Build history of the part. All positions in model axes, mm. Face numbers are marked on the shaded views. A direction names the side the tool comes from. Coordinates: 2 decimals unless noted, no trailing zeros. Write each loop counter-clockwise with the first axis right and the second up, starting at its lowest first coordinate (ties: lowest second). Pieces come first, ordered by that corner, then holes.
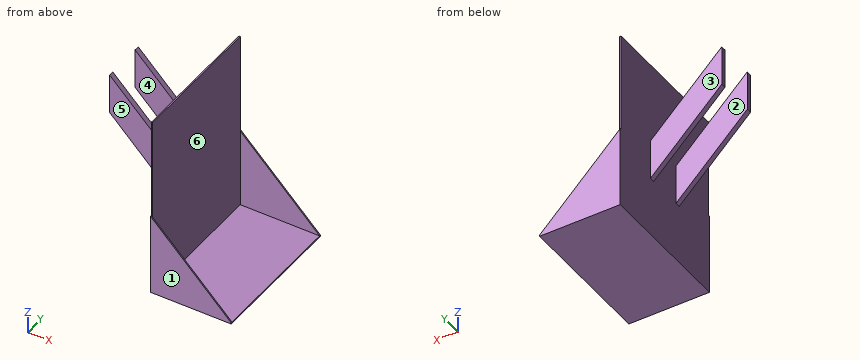
```python
from build123d import *

# Parameters (mm, degrees)
F0_W     = 101.6
F0_H     = 177.8
F1_DEPTH = 1.5875
F3_DEPTH = 1.5875
F5_DEPTH = 1.5875
F7_DEPTH = 1.5875
F8_W     = 6.35
F8_H     = 50.8


with BuildPart() as f1:
    # F0 (on Top) → F1 (new body)
    with BuildSketch(Plane.XY):
        with Locations((50.8, 88.9)):
            Rectangle(F0_W, F0_H)
    extrude(amount=F1_DEPTH)

    # F2 (on Front) → F3 (join)
    with BuildSketch(Plane.XZ):
        Polygon((0, 103.1875), (0, 1.5875), (101.6, 1.5875), align=None)
    extrude(amount=-F3_DEPTH)

    # F4 (on face) → F5 (join)
    with BuildSketch(Plane(origin=(0, 177.8, 0), x_dir=(-1, 0, 0), z_dir=(0, 1, 0))):
        Polygon((-101.6, 1.5875), (0, 1.5875), (0, 103.1875), align=None)
    extrude(amount=-F5_DEPTH)

    # F6 (on face) → F7 (join)
    with BuildSketch(Plane(origin=(0, 0, 0), x_dir=(0, -1, 0), z_dir=(-1, 0, 0))):
        Polygon((-176.2125, 1.5875), (-1.5875, 1.5875), (-1.5875, 103.1875), (-1.5875, 230.1875), (-176.2125, 230.1875), (-176.2125, 103.1875), align=None)
    extrude(amount=-F7_DEPTH)

    # F11: sweep along a path in F10
    with BuildLine(Plane(origin=(0, 66.675, 0), x_dir=(-1, 0, 0), z_dir=(0, 1, 0))) as f11_path:
        Line((0, 76.2), (89.8025612107, 166.0025612107))
    # F8 (on face) → F11 (sweep)
    with BuildSketch(Plane(origin=(0, 0, 0), x_dir=(0, -1, 0), z_dir=(-1, 0, 0))):
        with Locations((-63.5, 101.6)):
            Rectangle(F8_W, F8_H)
        with Locations((-114.3, 101.6)):
            Rectangle(F8_W, F8_H)
    sweep(path=f11_path.line)


solid = f1.part
```
1. Saw through at C-C on y = 16. List the corners of the cut face in (x, z).
Computed values:
outline: (0, 0) - (101.6, 0) - (101.6, 1.59) - (1.59, 1.59) - (1.59, 230.19) - (0, 230.19) - close
2. 3-axis set-ups, long thin cutter, end or side, ignore diameter. For the marked faces 4, 5 and 6: which of +Z, -Z, +X, -X, +Y, -Y reach the whole face in a straight line?
Computed values:
face 4: +Z, -Z, -X
face 5: +Z, -Z, -X, -Y
face 6: +Z, +X
3. Saw through at A-A on z = 133. List the corners of the cut face in (x, y) (1 decimal), plus the area to 3 significant figures.
Computed values:
outline: (-56.8, 60.3) - (-6, 60.3) - (-6, 66.7) - (-56.8, 66.7) - close; (-56.8, 111.1) - (-6, 111.1) - (-6, 117.5) - (-56.8, 117.5) - close; (0, 1.6) - (1.6, 1.6) - (1.6, 176.2) - (0, 176.2) - close
area: 922 mm2
4. Flat gauge pins, fed straight in: pin 1 (1 mm diameter, centred on y = 137.5, z = 80, fed in from -X); pin 2 (5 mm diameter, centred on x = -50.5, z = 164.5, fed in from -Y) (3 decimals); pin 3 (0.5 mm diameter, centred on x = 0.5, z = 143.5, fed in from -Y). Where does each tip first touch, or does it go through?
Computed values:
pin 1: stops at x = 0
pin 2: stops at y = 60.325
pin 3: stops at y = 1.59
5. Saw through at D-D on z = 209.5. List the corners of the cut face in (x, y) (1 decimal).
Computed values:
outline: (-89.8, 60.3) - (-82.5, 60.3) - (-82.5, 66.7) - (-89.8, 66.7) - close; (-89.8, 111.1) - (-82.5, 111.1) - (-82.5, 117.5) - (-89.8, 117.5) - close; (0, 1.6) - (1.6, 1.6) - (1.6, 176.2) - (0, 176.2) - close
6. Mould opens along Y. For the marked faces 1, 2 and 3 say: +Y half, -Y half, draft (parallel to the pull), parting line (faces both ways), or undercut.
Computed values:
face 1: -Y half
face 2: undercut
face 3: +Y half
7. Probe line 1 along Y through (x, z) = (24, 75); line 2 along Y through (x, z) = (-31, 117.5) (3 decimals); line 3 along X through (y, z) = (14, 100). List the from-to ranges inside material, lowest first.
Computed values:
line 1: y = 0 to 1.59, 176.21 to 177.8
line 2: y = 60.325 to 66.675, 111.125 to 117.475
line 3: x = 0 to 1.59
8. Saw through at B-B on x = -33. List the corners of the cut face in (y, z) (3 decimals), plus the area to 3 significant figures.
Computed values:
outline: (60.325, 109.2) - (66.675, 109.2) - (66.675, 160) - (60.325, 160) - close; (111.125, 109.2) - (117.475, 109.2) - (117.475, 160) - (111.125, 160) - close
area: 645 mm2
